Part model, mm, in its own coordinate system. A direction names the side the tool comes from. Coordinates: 2 decimals unless noted, no trailing zeros. Loops run counter-clockwise (first coordinate to the right, second up) from the corner with the lowest first, then second, coordinate; pieces in that order, holes last. Notation, with made-up numbers: M -31.75,0 L -18.75,0 A22 ccw -18.75,35 Z; hole C 61.5,-12 d7. An arc over 180 degrees is marked long. Use CSV: the item, a comma, the result in double quotes. Start each with the question number.
from build123d import *

# Parameters (mm, degrees)
FILLET1_R          = 10
SKETCH6_R          = 1.15
CUT_EXTRUDE1_DEPTH = 10


with BuildPart() as part:
    # Sketch2 → Revolve1 (revolve)
    with BuildSketch(Plane.XY, mode=Mode.PRIVATE) as revolve1_sk:
        Polygon((0, 4), (-2.43, 4), (-2.43, 3), (-2.43, 0), (-4.43, 0), (-4.43, 4), (-29.5, 4), (-29.5, 0), (-31.5, 0), (-31.5, 4), (-31.5, 6), (0, 6), align=None)
    revolve(revolve1_sk.sketch.rotate(Axis((0, 0, 0), (0, 1, 0)), 270), axis=Axis((0, 0, 0), (0, 1, 0)))

    # Fillet1
    # the kernel refuses this fillet: 10 mm, written as the material it adds along each edge
    with BuildSketch(Plane(origin=(0, 4, 0), x_dir=(0, 0, -1), z_dir=(1, 0, 0))) as fillet1_piece_1:
        with BuildLine():
            CenterArc((21.5, -10), FILLET1_R, 36.869897646, 53.130102354)
            Line((29.5, -4), (29.66, -3.88))
            ThreePointArc((29.66, -3.88), (29.7, -2), (29.7, 0))
            Line((29.7, 0), (29.5, 0.2))
            Line((29.5, 0.2), (21.5, 0.2))
            Line((21.5, 0.2), (21.5, 0))
        make_face()
    revolve(axis=Axis((0, 4, 0), (0, 1, 0)))
    with BuildSketch(Plane(origin=(0, 4, 0), x_dir=(0, 0, -1), z_dir=(1, 0, 0))) as fillet1_piece_2:
        with BuildLine():
            CenterArc((12.43, -10), FILLET1_R, 90, 53.130102354)
            Line((12.43, 0), (12.43, 0.2))
            Line((12.43, 0.2), (4.43, 0.2))
            Line((4.43, 0.2), (4.23, 0))
            ThreePointArc((4.23, 0), (4.23, -2), (4.27, -3.88))
            Line((4.27, -3.88), (4.43, -4))
        make_face()
    revolve(axis=Axis((0, 4, 0), (0, 1, 0)))

    # Sketch6 → Cut-Extrude1 (cut)
    with BuildSketch(Plane(origin=(0, 6, 0), x_dir=(1, 0, 0), z_dir=(0, 1, 0))):
        with Locations(Location((-11.275, 16.4, 0), (0, 0, 270))):
            Circle(SKETCH6_R)
        with Locations(Location((-11.275, -16.4, 0), (0, 0, 270))):
            Circle(SKETCH6_R)
    extrude(amount=-CUT_EXTRUDE1_DEPTH, mode=Mode.SUBTRACT)


solid = part.part
1. Pin check, flat tips, straight feed: pin 1 (3 mm diameter, centred on y = 4.5, z = -17.5, fed in from -X); pin 2 (5 mm diameter, centred on x = 14, z = -21, fed in from -Y); pin 3 (8 mm diameter, centred on x = 17, z = -21.5, fed in from -Y); pin 4 (1.5 mm diameter, centred on x = 14.5, y = 2, fed in from -Z). Stop position of each tip, or through.
2. Two-plate mould, pull along Z, no slides. Class faces 1 (the face through (-31.232, 2.958, 4.101)), 2 (the face through (0, 6, 0)), 3 (the face through (0, 4, 0)), 4 (the face through (1.479, 2.028, 1.928)): pulls with the +Z half, pulls with the -Z half, needs draft (parallel to the pull), parting line crosses it, or undercut.
3. Tool access for faces 5 (the face through (2, 0, 2)), 6 (the face through (9, 4, 9)): list every direction of +Z, -Z, +X, -X, +Y, -Y with a clear straight run to the whole face (end or side of a thin tool).
4. Slice it at C-C, the plane x = 0. List the corners of the cut face in (y, z).
5. Wall check: probe 1 along X at (y, z) = (1.4, -3.5); probe 2 along Y at (x, z) = (18.5, -4.5); probe 3 along X at (y, z) = (1.15, 0). Give the ranges that are in metal, low to high.
6. Slice it at A-A, the plane z = 0. List the corners of the cut face in (x, y).
7. Slice it at B-B, the plane y = 3.1. List the corners of the cut face in (x, z), and give its area (3 significant figures).
Found:
1,pin 1,"x = -27.13"
1,pin 2,"y = 1.82"
1,pin 3,"y = 0"
1,pin 4,"z = -28.34"
2,face 1,"parting line crosses it"
2,face 2,"needs draft"
2,face 3,"undercut"
2,face 4,"undercut"
3,face 5,"+Z, -Z, +X, -X, -Y"
3,face 6,"-Y"
4,outline,"M 0,-31.5 L 6,-31.5 L 6,31.5 L 0,31.5 L 0,29.5 A10 cw 4,21.5 L 4,12.43 A10 cw 0,4.43 L 0,2.43 L 4,2.43 L 4,-2.43 L 0,-2.43 L 0,-4.43 A10 cw 4,-12.43 L 4,-21.5 A10 cw 0,-29.5 Z"
5,probe 1,"-31.3 to -28.01, -4.5 to 4.5, 28.01 to 31.3"
5,probe 2,"4 to 6"
5,probe 3,"-31.5 to -28.49, -5.44 to -2.43, 2.43 to 5.44, 28.49 to 31.5"
6,outline,"M -31.5,0 L -29.5,0 A10 cw -21.5,4 L -12.43,4 A10 cw -4.43,0 L -2.43,0 L -2.43,4 L 2.43,4 L 2.43,0 L 4.43,0 A10 cw 12.43,4 L 21.5,4 A10 cw 29.5,0 L 31.5,0 L 31.5,6 L -31.5,6 Z"
7,outline,"C 0,0 d63; C 0,0 d16.57; hole C 0,0 d51.29; hole C 0,0 d4.86"
7,area,"1,250 mm^2"
